Source: CAD feature listing. Evaluate the final solid. Frame: model axes, mm. Give positions to 0.01 mm unless a question says otherwise; leave off trailing zeros. Write each loop counter-clockwise with the first axis right and the second up, starting at its lowest first coordinate (ties: lowest second). Pieces come first, ordered by that corner, then holes. Notation, with made-up numbers: (46, -33.5) - (61, -33.5) arc R13 cw to (61, -25.5) - close; hole circle Ø10 at (85, 76.25). An arc over 180 degrees is marked (long way). One line per question, with ' | ' between items. Start each with the question number.
(1) Section C-C, the plane z = 17.5. Return loops of the section in (x, y), plus the area to 3 significant figures.
(2) Ray query, line 1 (Z direction, x = 0, y = 0.6); line 2 (Z direction, x = 5.5, y = 0.25); line 3 (X direction, y = -1.55, z = 5.5). Return the intervals inside material, ascending. Write a range as [from, to].
(3) Section B-B, the plane z = 31.75. Return loops of the section in (x, y).
(4) Section A-A, the plane x = 0. Return loops of the section in (y, z).
(5) Pin query (flat end, axial travel): pin 1 (1.5 mm diameter, centred on x = 5.5, y = 2, fed in from -Z); pin 2 (2 mm diameter, centred on y = -2, z = 15, fed in from -X); pin 3 (2.5 mm diameter, centred on x = -28.5, y = -0.5, fed in from +Z). Return the tip coordinate at first contact, or that it passes through.
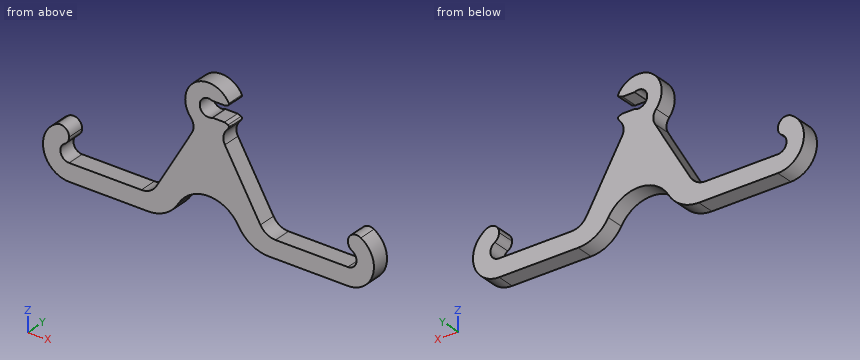
```python
from build123d import *

# Parameters (mm, degrees)
F1_DEPTH    = 2.38125
F2_DEPTH    = 2.38125
F3_T1_DEPTH = 6.5449897521
F3_T3_DEPTH = 6.5449897521
F4_T1_DEPTH = 13.0899795043
F5_R        = 0.396875
F6_R        = 3.175
F7_R        = 2.38124
F9_DEPTH    = 4.7635
F10_R       = 9.52499


# Not quite as in the source:
# - a fillet or chamfer that OpenCascade refuses, or shapes differently, is made with other operations: its cross-section is extruded or revolved along the edge and cut away or added
# - a fillet or chamfer is up to 0.001 mm smaller than in the source, because OpenCascade refuses the exact size


with BuildPart() as f1:
    # F0 (on Front) → F1 (new body, symmetric)
    with BuildSketch(Plane.XZ):
        with BuildLine():
            ThreePointArc((-38.1, 14.2875), (-45.24375, 7.14375), (-38.1, 0))
            Line((-38.1, 0), (38.1, 0))
            ThreePointArc((38.1, 0), (45.24375, 7.14375), (38.1, 14.2875))
            Line((38.1, 14.2875), (38.1, 9.525))
            ThreePointArc((38.1, 9.525), (40.48125, 7.14375), (38.1, 4.7625))
            Line((38.1, 4.7625), (18.3308710468, 4.7625))
            ThreePointArc((18.3308710468, 4.7625), (15.9496210468, 5.4005540145), (14.2064250612, 7.14375))
            Line((14.2064250612, 7.14375), (3.175, 26.250738686))
            ThreePointArc((3.175, 26.250738686), (0, 25.4), (-3.175, 26.250738686))
            Line((-3.175, 26.250738686), (-14.2064250612, 7.14375))
            ThreePointArc((-14.2064250612, 7.14375), (-15.9496210468, 5.4005540145), (-18.3308710468, 4.7625))
            Line((-18.3308710468, 4.7625), (-38.1, 4.7625))
            ThreePointArc((-38.1, 4.7625), (-40.48125, 7.14375), (-38.1, 9.525))
            Line((-38.1, 9.525), (-38.1, 14.2875))
        make_face()
    extrude(amount=F1_DEPTH, both=True)

    # F0 (on Front) → F2 (join, symmetric)
    with BuildSketch(Plane.XZ):
        with BuildLine():
            ThreePointArc((5.9830851103, 33.87725), (-4.0635273104, 36.6295743459), (-3.175, 26.250738686))
            ThreePointArc((-3.175, 26.250738686), (0, 25.4), (3.175, 26.250738686))
            ThreePointArc((3.175, 26.250738686), (4.8795743459, 27.6864726896), (5.9830851103, 29.62275))
            Line((5.9830851103, 29.62275), (1.0701210212, 29.62275))
            ThreePointArc((1.0701210212, 29.62275), (-2.38125, 31.75), (1.0701210212, 33.87725))
            Line((1.0701210212, 33.87725), (5.9830851103, 33.87725))
        make_face()
    extrude(amount=F2_DEPTH, both=True)

    # F3: chamfer of 0.396875 x 1.5875 on 2 edges, made by hand

    # F3_s2 → F3_t1 (cut)
    with BuildSketch(Plane.XZ):
        with BuildLine():
            Line((5.8436173462, 34.3923519359), (4.3177222428, 33.8561996981))
            Line((4.3177222428, 33.8561996981), (4.3177222428, 33.8244496981))
            ThreePointArc((4.3177222428, 33.8244496981), (5.1504036766, 33.8455), (5.9830851103, 33.8455))
            Line((5.9830851103, 33.8455), (6.0130005359, 33.88788625))
            ThreePointArc((6.0130005359, 33.88788625), (5.918565904, 34.1369039994), (5.872535886, 34.405458444))
            Line((5.872535886, 34.405458444), (5.8436173462, 34.3923519359))
        make_face()
    extrude(amount=F3_T1_DEPTH, mode=Mode.SUBTRACT)

    # F3_s4 → F3_t3 (cut)
    with BuildSketch(Plane.XZ.offset(-6.5449897521)):
        with BuildLine():
            Line((5.8436173462, 34.3923519359), (4.3177222428, 33.8561996981))
            Line((4.3177222428, 33.8561996981), (4.3177222428, 33.8244496981))
            ThreePointArc((4.3177222428, 33.8244496981), (5.1504036766, 33.8455), (5.9830851103, 33.8455))
            Line((5.9830851103, 33.8455), (6.0130005359, 33.88788625))
            ThreePointArc((6.0130005359, 33.88788625), (5.918565904, 34.1369039994), (5.872535886, 34.405458444))
            Line((5.872535886, 34.405458444), (5.8436173462, 34.3923519359))
        make_face()
    extrude(amount=F3_T3_DEPTH, mode=Mode.SUBTRACT)

    # F4: chamfer of 1.5875 x 0.396875 on 1 edges, made by hand

    # F4_s2 → F4_t1 (cut)
    with BuildSketch(Plane.XZ.offset(-6.5449897521)):
        with BuildLine():
            Line((4.3177222428, 29.6438003019), (5.8436173462, 29.1076480641))
            Line((5.8436173462, 29.1076480641), (5.872535886, 29.094541556))
            ThreePointArc((5.872535886, 29.094541556), (5.918565904, 29.3630960006), (6.0130005359, 29.61211375))
            Line((6.0130005359, 29.61211375), (5.9830851103, 29.6545))
            ThreePointArc((5.9830851103, 29.6545), (5.1504036766, 29.6545), (4.3177222428, 29.6755503019))
            Line((4.3177222428, 29.6755503019), (4.3177222428, 29.6438003019))
        make_face()
    extrude(amount=F4_T1_DEPTH, mode=Mode.SUBTRACT)

    # F5
    f5_edges = [f1.edges().sort_by_distance(p)[0] for p in [
        (5.783708, 0, 34.371302),
        (5.783708, 0, 29.128698),
        (1.070121, 0, 29.62275),
        (1.070121, 0, 33.87725),
    ]]
    fillet(f5_edges, radius=F5_R)

    # F6
    f6_edges = [f1.edges().sort_by_distance(p)[0] for p in [
        (3.175, 0, 26.250739),
        (-3.175, 0, 26.250739),
    ]]
    fillet(f6_edges, radius=F6_R)

    # F7 (radius 2.38125 in the source; OpenCascade refuses exactly that, so slightly less here)
    f7_edges = [f1.edges().sort_by_distance(p)[0] for p in [
        (38.1, 0, 14.2875),
        (38.1, 0, 9.525),
        (-38.1, 0, 14.2875),
        (-38.1, 0, 9.525),
    ]]
    fillet(f7_edges, radius=F7_R)

    # F8 (on face) → F9 (cut, through all)
    with BuildSketch(Plane.XZ.offset(2.38125)):
        Polygon((10.9985226281, 0), (0, 19.05), (-10.9985226281, 0), align=None)
    extrude(amount=-F9_DEPTH, mode=Mode.SUBTRACT)

    # F10 (radius 9.525 in the source; OpenCascade refuses exactly that, so slightly less here)
    f10_edges = [f1.edges().sort_by_distance(p)[0] for p in [
        (0, 0, 19.05),
        (10.998523, 0, 0),
        (-10.998523, 0, 0),
    ]]
    fillet(f10_edges, radius=F10_R)


solid = f1.part
```
Check sheet entries:
1) outline: (-8.23, -2.38) - (8.23, -2.38) - (8.23, 2.38) - (-8.23, 2.38) - close | area: 78.4 mm²
2) line 1: [9.53, 29.37], [34.13, 38.1] | line 2: [7.78, 22.22], [28.58, 29.19], [34.31, 34.92] | line 3: [-45.05, -39.82], [-15.79, -7.78], [7.78, 15.79], [39.82, 45.05]
3) outline: (-6.35, -2.38) - (-2.38, -2.38) - (-2.38, 2.38) - (-6.35, 2.38) - close
4) outline: (-2.38, 9.53) - (2.38, 9.53) - (2.38, 29.37) - (-2.38, 29.37) - close; (-2.38, 34.13) - (2.38, 34.13) - (2.38, 38.1) - (-2.38, 38.1) - close
5) pin 1: z = 7.19 | pin 2: x = -10.25 | pin 3: z = 4.76
